from build123d import *

# Parameters (mm, degrees)
SKETCH2_W              = 63.5
SKETCH2_H              = 15.875
BOSS_EXTRUDE1_DEPTH    = 15.875
F_1_4_20_TAPPED_HOLE_D = 5.1054
F_1_4_CLEARANCE_HOLE_D = 6.5278


with BuildPart() as part:
    # Sketch2 → Boss-Extrude1 (new body)
    with BuildSketch(Plane(origin=(0, 0, 0), x_dir=(1, 0, 0), z_dir=(0, 1, 0))):
        Rectangle(SKETCH2_W, SKETCH2_H)
    extrude(amount=-BOSS_EXTRUDE1_DEPTH)

    # 1/4-20 Tapped Hole (through all)
    with Locations(Plane(origin=(0, 0, 0), x_dir=(1, 0, 0), z_dir=(0, 1, 0))):
        with Locations((-10.16, 1.5875), (22.86, 1.5875)):
            Hole(F_1_4_20_TAPPED_HOLE_D / 2)

    # 1/4 Clearance Hole (through all)
    with Locations(Plane.XY.offset(7.9375)):
        with Locations((-22.86, -7.9375), (10.16, -7.9375)):
            Hole(F_1_4_CLEARANCE_HOLE_D / 2)


solid = part.part
Geometry: final body of the model. Coordinates: model frame, mm. Give positions to 0.01 mm unless a question says otherwise; leave off trailing zeros. Write each loop counter-clockwise with the first axis right and the second up, starting at its lowest first coordinate (ties: lowest second). Pieces come first, ordered by that corner, then holes. Notation, with made-up numbers: (12.25, -6.75) - (71.25, -6.75) arc R12 cw to (71.25, 2.25) - close; hole circle Ø11 at (75, -24.75). An arc over 180 degrees is marked (long way). Return JSON: item names as keys, results as strings. Group by question number.
1) Section C-C on y = -5.25. Return the cut outline in (x, z), plus the area to 3 significant figures.
2) Line query: line 1 (X direction, y = -8, z = 6.5); line 2 (X direction, y = -5.5, z = 6.75); line 3 (X direction, y = -10, z = -0.5). Output: solid intervals per line, ascending.
3) Section A-A on z = -0.5. State how many separate pieces and enclosed holes the cut face has, plus the area to 3 significant figures.
4) Mould query, pull axis Y, two halves, no side actions, for faces 1 (the flat face through (0, 0, 0)), 2 (the cylindrical face through (-8.134, -8.049, -0.034)), 3 (the cylindrical face through (-25.973, -6.957, -0.111)). Classes: released by +Y, released by -Y, zero draft, split by the parting line, or undercut.
5) Section B-B on x = -22.86. Return the cut outline in (y, z) (1 decimal), plus the area to 3 significant figures.
Filled in:
{
 "1": {"outline": "(-31.75, -7.94) - (-24.71, -7.94) - (-24.71, 7.94) - (-31.75, 7.94) - close; (-21.01, -7.94) - (8.31, -7.94) - (8.31, 7.94) - (-21.01, 7.94) - close; (12.01, -7.94) - (31.75, -7.94) - (31.75, 7.94) - (12.01, 7.94) - close; hole circle Ø5.11 at (-10.16, -1.59); hole circle Ø5.11 at (22.86, -1.59)", "area": "850 mm^2"},
 "2": {"line 1": "x = -31.75 to -26.12, -19.6 to 6.9, 13.42 to 31.75", "line 2": "x = -31.75 to -25.03, -20.69 to 7.99, 12.33 to 31.75", "line 3": "x = -31.75 to -25.39, -20.33 to -12.47, -7.85 to 7.63, 12.69 to 20.55, 25.17 to 31.75"},
 "3": {"separate pieces": "3", "enclosed holes": "2", "area": "794 mm^2"},
 "4": {"face 1": "released by +Y", "face 2": "zero draft", "face 3": "undercut"},
 "5": {"outline": "(-15.9, -7.9) - (-11.2, -7.9) - (-11.2, 7.9) - (-15.9, 7.9) - close; (-4.7, -7.9) - (0, -7.9) - (0, 7.9) - (-4.7, 7.9) - close", "area": "148 mm^2"}
}
